```python
from build123d import *

# Parameters (mm, degrees)
BOSS_EXTRU_1_DEPTH                                = 30
ENL_V_MAT_EXTRU_1_DEPTH                           = 15
BOSS_EXTRU_2_DEPTH                                = 10
BOSS_EXTRU_3_DEPTH                                = 10
BOSS_EXTRU_4_DEPTH                                = 10
BOSS_EXTRU_5_DEPTH                                = 10
DIAM_TRE_DU_PER_AGE_4_2_4_2_1_D                   = 4.2
DIAM_TRE_DU_PER_AGE_4_2_4_2_1_DEPTH               = 40
CHAMBRAGE_POUR_VIS_T_TE_HEXAGONALE_M3_D           = 4.2
CHAMBRAGE_POUR_VIS_T_TE_HEXAGONALE_M3_DEPTH       = 40
CHAMBRAGE_POUR_VIS_T_TE_HEXAGONALE_M3_CBORE_D     = 20
CHAMBRAGE_POUR_VIS_T_TE_HEXAGONALE_M3_CBORE_DEPTH = 15
CONG_1_R                                          = 10
CONG_2_R                                          = 20
ENL_V_MAT_EXTRU_2_DEPTH                           = 270.645454496
TROU_TARAUD_M5X0_81_D                             = 4.2
TROU_TARAUD_M5X0_81_ON_FACE_2_D                   = 4.2
BOSS_EXTRU_6_DEPTH                                = 15
ESQUISSE14_W                                      = 344.623968027
ESQUISSE14_H                                      = 364.856294917
ENL_V_MAT_EXTRU_3_DEPTH                           = 12
BOSS_EXTRU_7_DEPTH                                = 15
ESQUISSE16_W                                      = 47
ESQUISSE16_H                                      = 54.5
ENL_V_MAT_EXTRU_4_DEPTH                           = 12
ESQUISSE17_R                                      = 0.5
ENL_V_MAT_EXTRU_5_DEPTH                           = 12
TROU_TARAUD_M2_2X0_451_D                          = 1.75
ENL_V_MAT_EXTRU_6_DEPTH                           = 270.645454496
BOSS_EXTRU_8_DEPTH                                = 15
ESQUISSE21_W                                      = 34.017882368
ESQUISSE21_H                                      = 54.5
ENL_V_MAT_EXTRU_7_DEPTH                           = 12
TROU_TARAUD_M5X0_82_D                             = 4.2
TROU_TARAUD_M5X0_82_DEPTH                         = 54.927
TROU_TARAUD_M5X0_82_TIP                           = 1.2618073
TROU_TARAUD_M5X0_84_D                             = 4.2
TROU_TARAUD_M5X0_84_DEPTH                         = 54.927
TROU_TARAUD_M5X0_84_TIP                           = 1.2618073


with BuildPart() as part:
    # Esquisse1 → Boss.-Extru.1 (new body)
    with BuildSketch(Plane.XY.offset(30)):
        Polygon((33.943844834, -122.117785393), (33.943844834, 157.882214607), (-206.056155166, 157.882214607), (-206.056155166, -122.117785393), (-179.056155166, -162.614832092), (-152.268878217, -162.614832092), (-139.750990012, -172.117785393), (-32.361320321, -172.117785393), (-19.843432116, -162.614832092), (6.943844834, -162.614832092), align=None)
    extrude(amount=-BOSS_EXTRU_1_DEPTH)

    # Esquisse2 → Enlèv. mat.-Extru.1 (cut)
    with BuildSketch(Plane.XY.offset(30)):
        Polygon((-123.206083599, 157.882214607), (-123.206083599, 147.882214607), (-190.556155166, 147.882214607), (-190.556155166, -121.431981452), (-173.70399548, -146.708377667), (-152.268878217, -146.708377667), (-140.175798707, -146.685066621), (-133.019479604, -152.117785393), (-39.092830728, -152.117785393), (-31.936511626, -146.685066621), (-19.843432116, -146.708377667), (1.141061448, -146.708377667), (18.443844834, -122.117785393), (18.443844834, 147.882214607), (-48.906226734, 147.882214607), (-48.906226734, 157.882214607), align=None)
    extrude(amount=-ENL_V_MAT_EXTRU_1_DEPTH, mode=Mode.SUBTRACT)

    # Esquisse3 → Boss.-Extru.2 (add)
    with BuildSketch(Plane(origin=(0, 0, 0), x_dir=(-1, 0, 0), z_dir=(0, 0, -1))):
        Polygon((162.596079372, 137.882214607), (162.596079372, 147.882214607), (190.556155166, 147.882214607), (190.556155166, 118.944465923), (180.556155166, 118.944465923), (180.556155166, 137.882214607), align=None)
    extrude(amount=BOSS_EXTRU_2_DEPTH)

    # Esquisse4 → Boss.-Extru.3 (add)
    with BuildSketch(Plane(origin=(0, 0, 0), x_dir=(-1, 0, 0), z_dir=(0, 0, -1))):
        Polygon((152.268878217, -136.708377667), (168.352374382, -136.708377667), (180.556155166, -118.404041358), (190.556155166, -121.431981452), (173.70399548, -146.708377667), (152.268878217, -146.708377667), align=None)
    extrude(amount=BOSS_EXTRU_3_DEPTH)

    # Esquisse5 → Boss.-Extru.4 (add)
    with BuildSketch(Plane(origin=(0, 0, 0), x_dir=(-1, 0, 0), z_dir=(0, 0, -1))):
        Polygon((-8.443844834, 137.882214607), (-8.443844834, 118.944465923), (-18.443844834, 118.944465923), (-18.443844834, 147.882214607), (9.516230961, 147.882214607), (9.516230961, 137.882214607), align=None)
    extrude(amount=BOSS_EXTRU_4_DEPTH)

    # Esquisse6 → Boss.-Extru.5 (add)
    with BuildSketch(Plane(origin=(0, 0, 0), x_dir=(-1, 0, 0), z_dir=(0, 0, -1))):
        Polygon((3.759935951, -136.708377667), (19.843432116, -136.708377667), (19.843432116, -146.708377667), (-1.141061448, -146.708377667), (-18.443844834, -122.117785393), (-8.443844834, -118.404041358), align=None)
    extrude(amount=BOSS_EXTRU_5_DEPTH)

    # Diamètre du perçage Ø4.2 (4.2)1
    with Locations(Plane.XY.offset(30)):
        with Locations((26.438895769, -119.607785393), (-198.551206101, -119.607785393)):
            Hole(DIAM_TRE_DU_PER_AGE_4_2_4_2_1_D / 2, depth=DIAM_TRE_DU_PER_AGE_4_2_4_2_1_DEPTH)

    # Chambrage pour vis à tête hexagonale M3.51
    with Locations(Plane.XY.offset(30)):
        with Locations((-199.94021721, 151.76627665), (27.827906877, 151.76627665)):
            CounterBoreHole(CHAMBRAGE_POUR_VIS_T_TE_HEXAGONALE_M3_D / 2, CHAMBRAGE_POUR_VIS_T_TE_HEXAGONALE_M3_CBORE_D / 2, CHAMBRAGE_POUR_VIS_T_TE_HEXAGONALE_M3_CBORE_DEPTH, depth=CHAMBRAGE_POUR_VIS_T_TE_HEXAGONALE_M3_DEPTH)

    # Congé1
    cong_1_edges = [part.edges().sort_by_distance(p)[0] for p in [
        (8.443844834, 137.882214607, -5),
        (-180.556155166, 137.882214607, -5),
    ]]
    fillet(cong_1_edges, radius=CONG_1_R)

    # Congé2
    cong_2_edges = [part.edges().sort_by_distance(p)[0] for p in [
        (18.443844834, 147.882214607, -5),
        (18.443844834, 147.882214607, 22.5),
        (-190.556155166, 147.882214607, 22.5),
        (-190.556155166, 147.882214607, -5),
    ]]
    fillet(cong_2_edges, radius=CONG_2_R)

    # Esquisse11 → Enlèv. mat.-Extru.2 (cut, through all)
    with BuildSketch(Plane.XY.offset(15)):
        Polygon((-123.206083599, 147.882214607), (-123.206083599, 47.882214607), (-190.556155166, -22.43592162), (-190.556155166, -92.767969228), (18.443844834, -92.767969228), (18.443844834, -22.43592162), (-48.906226734, 47.882214607), (-48.906226734, 147.882214607), align=None)
        Polygon((-138.206083599, 147.882214607), (-138.206083599, 57.882214607), (-190.556155166, 3.225116578), (-190.556155166, 95.532143039), (-190.556155166, 104.207178823), (-146.881119383, 147.882214607), align=None)
        Polygon((-33.906226734, 57.882214607), (18.443844834, 3.225116578), (18.443844834, 95.532143039), (18.443844834, 104.207178823), (-25.23119095, 147.882214607), (-33.906226734, 147.882214607), align=None)
    extrude(amount=-ENL_V_MAT_EXTRU_2_DEPTH, mode=Mode.SUBTRACT)

    # Trou taraudé M5x0.81 (through all)
    with Locations(Plane(origin=(-199.94021721, 151.76627665, 15), x_dir=(1, 0, 0), z_dir=(0, 0, 1))):
        with Locations((0, 0), (227.768124087, 0)):
            Hole(TROU_TARAUD_M5X0_81_D / 2)

    # Trou taraudé M5x0.81 on face 2 (through all)
    with Locations(Plane(origin=(26.438895769, -119.607785393, 30), x_dir=(1, 0, 0), z_dir=(0, 0, 1))):
        with Locations((0, 0), (-224.99010187, 0)):
            Hole(TROU_TARAUD_M5X0_81_ON_FACE_2_D / 2)

    # Esquisse13 → Boss.-Extru.6 (add)
    with BuildSketch(Plane.XY.offset(15)):
        Polygon((-48.906226734, 47.882214607), (-123.206083599, 47.882214607), (-148.90605105, 21.049669812), (-190.556155166, -22.43592162), (-190.556155166, -49.268466414), (-123.206083599, 21.049669812), (-48.906226734, 21.049669812), (18.443844834, -49.268466414), (18.443844834, -22.43592162), (-23.206259282, 21.049669812), align=None)
    extrude(amount=-BOSS_EXTRU_6_DEPTH)

    # Esquisse14 → Enlèv. mat.-Extru.3 (cut)
    with BuildSketch(Plane.XY.offset(30)):
        with Locations((-76.951608065, -8.129401738)):
            Rectangle(ESQUISSE14_W, ESQUISSE14_H)
    extrude(amount=-ENL_V_MAT_EXTRU_3_DEPTH, mode=Mode.SUBTRACT)

    # Esquisse15 → Boss.-Extru.7 (add)
    with BuildSketch(Plane.XY.offset(15)):
        Polygon((-165.240705537, 11.949496673), (-165.240705537, -16.671939758), (-10.373483375, -16.671939758), (-10.373483375, 17.080639576), (-29.498652377, 36.205808578), (-140.984393632, 36.205808578), align=None)
    extrude(amount=-BOSS_EXTRU_7_DEPTH)

    # Esquisse16 → Enlèv. mat.-Extru.4 (cut)
    with BuildSketch(Plane.XY.offset(15)):
        with Locations((-86.056155166, 16.099315521)):
            Rectangle(ESQUISSE16_W, ESQUISSE16_H)
    extrude(amount=-ENL_V_MAT_EXTRU_4_DEPTH, mode=Mode.SUBTRACT)

    # Esquisse17 → Enlèv. mat.-Extru.5 (cut)
    with BuildSketch(Plane.XY.offset(3)):
        with Locations((-97.061155166, 40.869315521)):
            Circle(ESQUISSE17_R)
        with Locations((-65.141155166, 16.099315521)):
            Circle(ESQUISSE17_R)
        with Locations((-97.061155166, -8.670684479)):
            Circle(ESQUISSE17_R)
    extrude(amount=-ENL_V_MAT_EXTRU_5_DEPTH, mode=Mode.SUBTRACT)

    # Trou taraudé M2.2x0.451 (through all)
    with Locations(Plane(origin=(-97.061155166, 40.869315521, 3), x_dir=(1, 0, 0), z_dir=(0, 0, 1))):
        with Locations((0, 0), (31.92, -24.77), (0, -49.54)):
            Hole(TROU_TARAUD_M2_2X0_451_D / 2)

    # Esquisse19 → Enlèv. mat.-Extru.6 (cut, through all)
    with BuildSketch(Plane.XY.offset(15)):
        Polygon((-138.206083599, -92.767969228), (-138.206083599, -16.671939758), (-159.335498292, -16.671939758), (-190.556155166, -49.268466414), (-190.556155166, -92.767969228), align=None)
        Polygon((-190.556155166, 3.225116578), (-138.206083599, 57.882214607), (-190.556155166, 57.882214607), align=None)
        Polygon((-138.206083599, -16.671939758), (-138.206083599, 57.882214607), (-190.556155166, 3.225116578), (-190.556155166, -49.268466414), (-159.335498292, -16.671939758), align=None)
        Polygon((18.443844834, 57.882214607), (-33.906226734, 57.882214607), (18.443844834, 3.225116578), align=None)
        Polygon((-33.906226734, 57.882214607), (-33.906226734, -16.671939758), (-12.77681204, -16.671939758), (18.443844834, -49.268466414), (18.443844834, 3.225116578), align=None)
        Polygon((-12.77681204, -16.671939758), (-33.906226734, -16.671939758), (-33.906226734, -92.767969228), (18.443844834, -92.767969228), (18.443844834, -49.268466414), align=None)
    extrude(amount=-ENL_V_MAT_EXTRU_6_DEPTH, mode=Mode.SUBTRACT)

    # Esquisse20 → Boss.-Extru.8 (add)
    with BuildSketch(Plane.XY.offset(15)):
        Polygon((-138.206083599, -16.671939758), (-138.206083599, -97.039238238), (-123.206083599, -97.039238238), (-123.206083599, 49.892057072), (-138.206083599, 49.892057072), align=None)
        Polygon((-48.906226734, 49.892057072), (-33.906226734, 49.892057072), (-33.906226734, -16.671939758), (-33.906226734, -97.039238238), (-48.906226734, -97.039238238), align=None)
    extrude(amount=-BOSS_EXTRU_8_DEPTH)

    # Esquisse21 → Enlèv. mat.-Extru.7 (cut)
    with BuildSketch(Plane.XY.offset(15)):
        with Locations((-126.56509635, 16.099315521)):
            Rectangle(ESQUISSE21_W, ESQUISSE21_H)
    extrude(amount=-ENL_V_MAT_EXTRU_7_DEPTH, mode=Mode.SUBTRACT)

    # Trou taraudé M5x0.82
    with Locations(Plane(origin=(-130.206083599, 77.882214607, 15), x_dir=(1, 0, 0), z_dir=(0, 0, 1))):
        with Locations((0, 0), (88.299856865, 0)):
            Hole(TROU_TARAUD_M5X0_82_D / 2, depth=TROU_TARAUD_M5X0_82_DEPTH)
            with Locations((0, 0, -(TROU_TARAUD_M5X0_82_DEPTH + TROU_TARAUD_M5X0_82_TIP / 2))):  # 118° drill point
                Cone(0, TROU_TARAUD_M5X0_82_D / 2, TROU_TARAUD_M5X0_82_TIP, mode=Mode.SUBTRACT)

    # Trou taraudé M5x0.84
    with Locations(Plane(origin=(-130.206083599, -47.117785393, 15), x_dir=(1, 0, 0), z_dir=(0, 0, 1))):
        with Locations((0, 0), (88.299856865, 0)):
            Hole(TROU_TARAUD_M5X0_84_D / 2, depth=TROU_TARAUD_M5X0_84_DEPTH)
            with Locations((0, 0, -(TROU_TARAUD_M5X0_84_DEPTH + TROU_TARAUD_M5X0_84_TIP / 2))):  # 118° drill point
                Cone(0, TROU_TARAUD_M5X0_84_D / 2, TROU_TARAUD_M5X0_84_TIP, mode=Mode.SUBTRACT)


solid = part.part
```
Could you check a few things on this model? Use its own coordinates, in mm. A direction names the side the tool comes from. Round coordinates to 2 decimals unless told otherwise and drop trailing zeros. Write each loop counter-clockwise with the first axis right and the second up, starting at its lowest first coordinate (ties: lowest second). Pieces come first, ordered by that corner, then holes. Notation, with made-up numbers: M 83.25,55 L 113.25,55 A12 ccw 113.25,60 Z; hole C 52.25,87.25 d9. An arc over 180 degrees is marked long. Write each question's results on one line, items separated by ' | '. Start each with the question number.
1. Imagine slicing it at D-D on z = 9.5. Count the separate pieces of the cut face and the enclosed holes in it, and give its area (3 significant figures).
2. I need wall thicknesses on L1, parallel to X at y = -13, z = 1; L2, parallel to X at y = -86, z = 11.5; L3, parallel to Z at x = -179, y = -154.5. Which ranges of each line are inside material? Lowest first, please. Write a range as from..to.
3. Imagine slicing it at C-C on y = -109. List the corners of the cut face in (x, z) for me.
4. Imagine slicing it at A-A on y = -54. List the corners of the cut face in (x, z) for me, and give its area (3 significant figures).
5. On a 3-axis mill with a long thin cutter (end or side, diameter ignored), from which of +Z, -Z, +X, -X, +Y, -Y can I reach the whole of each face in a straight line? I mean faces 1 (the face through (-182.25, -133.89, 16.52)), 2 (the face through (-186, 118.944, -5)), 3 (the face through (-5, 147.882, -5)), 4 (the face through (-87, -92.768, 8)), 5 (the face through (-174.37, -127.68, -4.93)). Say none if no direction works.
6. Imagine slicing it at B-B on x = -117.5. List the corners of the cut face in (y, z) for me.
7. Thinking about a two-plate mould opening in Y: for faces 6 (the face through (-182.25, -133.89, -4.93)), 7 (the face through (-206.056, 20, 9)), 8 (the face through (-193.013, 144.554, 16.521)), 9 (the face through (-12, -136.708, -5)), which applies, +Y half, -Y half, draft (parallel to the pull), parting line (faces both ways), or undercut?
8. I'm going to push flat-ended pins straight in: pin 1 Ø6.5 at (x, y) = (27.83, 151.77) entering from -Z; pin 2 Ø11 at (y, z) = (-140.5, -4.5) entering from -X; pin 3 Ø8 at (x, y) = (-198, 152) entering from +Z. Where does each tip first touch, or does it pass through?
Result sheet:
1) separate pieces: 1 | enclosed holes: 12 | area: 36,400 mm^2
2) L1: x = -206.06..-190.56, -138.21..-33.91, 18.44..33.94 | L2: x = -206.06..-190.56, -138.21..-123.21, -48.91..-33.91, 18.44..33.94 | L3: z = 0..18
3) outline: M -206.06,0 L 33.94,0 L 33.94,18 L 18.44,18 L 18.44,15 L -190.56,15 L -190.56,18 L -206.06,18 Z
4) outline: M -206.06,0 L -190.56,0 L -190.56,18 L -206.06,18 Z; M -138.21,0 L -123.21,0 L -123.21,15 L -138.21,15 Z; M -48.91,0 L -33.91,0 L -33.91,15 L -48.91,15 Z; M 18.44,0 L 33.94,0 L 33.94,18 L 18.44,18 Z | area: 1,010 mm^2
5) face 1: +Z | face 2: -Z, +X, -X | face 3: -Z, +X, -X, +Y | face 4: +Z, -Z | face 5: -Z
6) outline: M -172.12,0 L -92.77,0 L -92.77,15 L -152.12,15 L -152.12,18 L -172.12,18 Z; M -16.67,0 L 47.88,0 L 47.88,15 L 43.35,15 L 43.35,3 L -11.15,3 L -11.15,15 L -16.67,15 Z; M 147.88,0 L 157.88,0 L 157.88,15 L 147.88,15 Z
7) face 6: -Y half | face 7: draft | face 8: undercut | face 9: undercut
8) pin 1: stops at z = 0 | pin 2: stops at x = -195.91 | pin 3: stops at z = 15
